Autodesk Inventor part; units mm, degrees
ref_plane "YZ Plane" through (0, 0, 0) normal (1, 0, 0) x (0, 1, 0)
ref_plane "XZ Plane" through (0, 0, 0) normal (0, 1, 0) x (-1, 0, 0)
ref_plane "XY Plane" through (0, 0, 0) normal (0, 0, 1) x (1, 0, 0)
sketch "Sketch1" plane through (0, 0, 0) normal (0, 0, 1) x (1, 0, 0)
  line L0 (0, 0) -> (160, 0)
  line L1 (160, 0) -> (118.589, 154.5481)
  line L2 (41.411, 154.5481) -> (0, 0)
  line L3 (41.411, 154.5481) -> (118.589, 154.5481)
  dimension "d0" = 160
  dimension "d1" = 160
  dimension "d2" = 75
  dimension "d8" = 75
extrude "Extrusion1" add sketch "Sketch1" along normal blind 55
sketch "Sketch7" plane through (0, 0, 0) normal (0, 0, -1) x (-1, 0, 0)
  circle A0 centre (-80, 304.672) radius 315 construction
  line L0 (0, 0) -> (-160, 0)
  arc A1 (-160, 0) -> (0, 0) centre (-80, 304.672) ccw
  dimension "d28" = 630
extrude "Extrusion6" add sketch "Sketch7" against normal blind 55
sketch "Sketch19" plane through (0, 0, 0) normal (0, 0, -1) x (-1, 0, 0)
  circle A0 centre (-80, 4.836) radius 10
  line L0 (-118.589, 154.5481) -> (-41.411, 154.5481)
  line L1 (-80, 154.5481) -> (-80, -10.328)
  arc A1 (-160, 0) -> (0, 0) centre (-80, 304.672) ccw
  dimension "d112" = 20
  dimension "d113" = 15.164
extrude "Extrusion19" cut sketch "Sketch19" against normal through all
sketch "Sketch20" plane through (0, 0, 0) normal (0, 0, -1) x (-1, 0, 0)
  line L0 (-41.411, 154.5481) -> (0, 0)
  circle A0 centre (-80, 4.836) radius 10
  line L1 (-41.411, 154.5481) -> (0, 0)
  line L2 (-118.589, 154.5481) -> (-41.411, 154.5481)
  line L3 (-160, 0) -> (-118.589, 154.5481)
  arc A1 (-160, 0) -> (0, 0) centre (-80, 304.672) ccw
  line L4 (-49.0843, 144.5481) -> (-12.3033, 7.2797)
  arc A2 (-147.6967, 7.2797) -> (-12.3033, 7.2797) centre (-80, 304.672) ccw
  line L5 (-147.6967, 7.2797) -> (-110.9157, 144.5481)
  line L6 (-110.9157, 144.5481) -> (-49.0843, 144.5481)
  line L7 (-15.6678, 19.836) -> (-144.3322, 19.836)
  dimension "d116" = 10
  dimension "d119" = 15
extrude "Extrusion20" cut sketch "Sketch20" against normal through all contours L5 L6 L4 L7
sketch "Sketch21" plane through (0, 0, 0) normal (0, 0, -1) x (-1, 0, 0)
  line L0 (-110.9157, 144.5481) -> (-49.0843, 144.5481)
  line L1 (-75, 144.5481) -> (-75, 19.836)
  line L2 (-15.6678, 19.836) -> (-144.3322, 19.836)
  line L3 (-85, 19.836) -> (-85, 144.5481)
  line L4 (-85, 144.5481) -> (-75, 144.5481)
  line L5 (-75, 19.836) -> (-85, 19.836)
  point P0 (0, 0)
  point P1 (-80, 144.5481)
  point P2 (-80, 144.5481)
  dimension "d120" = 10
extrude "Extrusion21" add sketch "Sketch21" against normal blind 55
sketch "Sketch22" plane through (0, 0, 0) normal (0, 0, -1) x (-1, 0, 0)
  line L0 (-15.6678, 19.836) -> (-49.0843, 144.5481)
  line L1 (-33.7158, 87.1921) -> (-126.2842, 87.1921)
  line L2 (-110.9157, 144.5481) -> (-144.3322, 19.836)
  line L3 (-80, 87.1921) -> (-80, 77.1921)
  line L4 (-31.0363, 77.1921) -> (-128.9637, 77.1921)
  line L5 (-75, 19.836) -> (-75, 144.5481)
  line L6 (-33.7158, 87.1921) -> (-31.0363, 77.1921)
  line L7 (-126.2842, 87.1921) -> (-128.9637, 77.1921)
  point P0 (0, 0)
  point P1 (-80, 82.1921)
  point P2 (-75, 82.1921)
  dimension "d124" = 10
extrude "Extrusion22" add sketch "Sketch22" against normal blind 55
sketch "Sketch23" plane through (0, 0, 0) normal (0, 0, -1) x (-1, 0, 0)
  circle A0 centre (-80, 60) radius 55
  line L0 (-118.589, 154.5481) -> (-41.411, 154.5481)
  line L1 (-57.5, 82.5) -> (-102.5, 82.5)
  line L2 (-102.5, 82.5) -> (-102.5, 37.5)
  line L3 (-102.5, 37.5) -> (-57.5, 37.5)
  line L4 (-57.5, 37.5) -> (-57.5, 82.5)
  point P0 (0, 0)
  point P1 (-80, 154.5481)
  point P2 (-102.5, 60)
  point P3 (-80, 82.5)
  dimension "d127" = 110
  dimension "d128" = 60
  dimension "d129" = 45
  dimension "d130" = 45
extrude "Extrusion23" cut sketch "Sketch23" against normal blind 30 contours L4 L3 L2 L1
sketch "Sketch24" plane through (118.589, 154.5481, 55) normal (0.9659, 0.2588, 0) x (0, 0, -1)
  line L0 (45.475, -9.525) -> (45.475, -150.475) construction
  line L1 (9.525, -150.475) -> (9.525, -9.525) construction
  line L2 (0, -160) -> (0, 0) construction
  circle A0 centre (45.475, -150.475) radius 2.5
  circle A1 centre (9.525, -150.475) radius 2.5
  circle A2 centre (9.525, -9.525) radius 2.5
  circle A3 centre (45.475, -9.525) radius 2.5
  circle A4 centre (18.4199, -150.475) radius 2.5
  circle A5 centre (36.5801, -150.475) radius 2.5
  circle A6 centre (36.5801, -9.525) radius 2.5
  circle A7 centre (18.4199, -9.525) radius 2.5
  point P0 (55, -118.589)
  point P1 (9.525, -80)
  point P2 (0, -80)
  dimension "d133" = 140.95
  dimension "d134" = 140.95
  dimension "d135" = 9.525
  dimension "d136" = 9.525
  dimension "d137" = 5
  dimension "d138" = 5
  dimension "d139" = 5
  dimension "d140" = 5
  dimension "d141" = 5
  dimension "d142" = 5
  dimension "d143" = 5
  dimension "d144" = 5
  dimension "d145" = 18.4199
  dimension "d146" = 18.4199
extrude "Extrusion24" cut sketch "Sketch24" against normal blind 25
sketch "Sketch25" plane through (41.411, 154.5481, 0) normal (-0.9659, 0.2588, 0) x (0, 0, 1)
  line L0 (45.475, -9.525) -> (45.475, -150.475) construction
  line L1 (9.525, -150.475) -> (9.525, -9.525) construction
  circle A0 centre (45.475, -150.475) radius 2.5
  circle A1 centre (9.525, -150.475) radius 2.5
  circle A2 centre (9.525, -9.525) radius 2.5
  circle A3 centre (45.475, -9.525) radius 2.5
  circle A4 centre (18.4199, -150.475) radius 2.5
  circle A5 centre (36.5801, -150.475) radius 2.5
  circle A6 centre (36.5801, -9.525) radius 2.5
  circle A7 centre (18.4199, -9.525) radius 2.5
  line L2 (0, 0) -> (0, -160)
  line L3 (55, 0) -> (55, -160)
  point P0 (9.525, -80)
  point P1 (0, -80)
  dimension "d149" = 140.95
  dimension "d150" = 140.95
  dimension "d153" = 5
  dimension "d154" = 5
  dimension "d155" = 5
  dimension "d156" = 5
  dimension "d157" = 5
  dimension "d158" = 5
  dimension "d159" = 5
  dimension "d160" = 5
  dimension "d163" = 9.525
  dimension "d164" = 18.4199
  dimension "d165" = 18.4199
  dimension "d166" = 9.525
extrude "Extrusion25" cut sketch "Sketch25" against normal blind 25
properties part number "CA001" material "ABS Plastic"
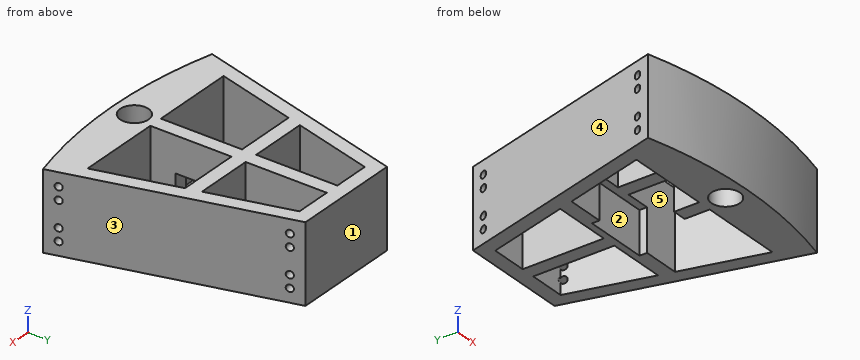
Model file for the job. Use its own axes, mm. Face numbers are marked on the shaded views. A direction names the side the tool comes from. Coordinates: 2 decimals unless noted, no trailing zeros. Write each loop counter-clockwise with the first axis right and the second up, starting at its lowest first coordinate (ties: lowest second). Pieces come first, ordered by that corner, then holes. Notation, with made-up numbers: (46.25, 0) - (55.25, 0) arc R23 cw to (55.25, 27) - close; hole circle Ø7 at (11, -40). An arc over 180 degrees is marked (long way). One line per item, written item: value. Start each with the question number.
1. Mould opens along X. For the marked faces 1, 2 and 3 say: released by +X, released by -X, zero draft, split by the parting line, or undercut.
2. Slice it at A-A (x = 80). Write the cut outline in (y, z), plus the area to 3 significant figures.
3. Slice it at D-D (x = 105.5). Write the cut outline in (y, z), plus the area to 3 significant figures.
4. Flat gauge pins, fed straight in: pin 1 (1.5 mm diameter, centred on y = 31.5, z = 29, fed in from -X); pin 2 (4 mm diameter, centred on x = 108, y = 18, fed in from -Z); pin 3 (6 mm diameter, centred on y = 59, z = 17.5, fed in from -X); pin 4 (13 mm diameter, centred on x = 97, z = 39, fed in from -Y). Where does each tip first touch, or does it go through?
5. Slice it at B-B (y = 47). Write the cut outline in (x, z).
6. Slice it at C-C (z = 4). Write the cut outline in (x, y).
7. Tool access for the marked faces 4 and 5: list every direction of +Z, -Z, +X, -X, +Y, -Y with a clear straight run to the whole face (end or side of a thin tool).
8. Probe line 1 (Y direction, x = 80, z = 17); line 2 (Y direction, x = 80, z = 34); line 3 (X direction, y = 109, z = 42). List the from-to ranges inside material, lowest first. Write a range as from..to.
Answers below:
1. face 1: zero draft
1. face 2: undercut
1. face 3: released by +X
2. outline: (-10.33, 0) - (-5.16, 0) - (-5.16, 55) - (-10.33, 55) - close; (14.84, 0) - (37.5, 0) - (37.5, 30) - (82.5, 30) - (82.5, 0) - (154.55, 0) - (154.55, 55) - (14.84, 55) - close
2. area: 6,620 mm^2
3. outline: (-9.29, 0) - (19.84, 0) - (19.84, 55) - (-9.29, 55) - close; (77.19, 0) - (87.19, 0) - (87.19, 55) - (77.19, 55) - close; (144.55, 0) - (154.55, 0) - (154.55, 55) - (144.55, 55) - close
3. area: 2,700 mm^2
4. pin 1: stops at x = 8.24
4. pin 2: stops at z = 0
4. pin 3: stops at x = 15.01
4. pin 4: stops at y = -10.15
5. outline: (12.59, 0) - (22.95, 0) - (22.95, 55) - (12.59, 55) - close; (75, 30) - (85, 30) - (85, 55) - (75, 55) - close; (137.05, 0) - (147.41, 0) - (147.41, 55) - (137.05, 55) - close
6. outline: (0, 0) arc R315 ccw to (160, 0) - (118.59, 154.55) - (41.41, 154.55) - close; hole (15.67, 19.84) - (75, 19.84) - (75, 37.5) - (85, 37.5) - (85, 19.84) - (144.33, 19.84) - (128.96, 77.19) - (102.5, 77.19) - (102.5, 82.5) - (57.5, 82.5) - (57.5, 77.19) - (31.04, 77.19) - close; hole (33.72, 87.19) - (75, 87.19) - (75, 144.55) - (49.08, 144.55) - close; hole circle Ø20 at (80, 4.84); hole (85, 87.19) - (126.28, 87.19) - (110.92, 144.55) - (85, 144.55) - close
7. face 4: +Z, -Z, -X, +Y
7. face 5: +Z, -Z
8. line 1: y = -10.33..-5.16, 14.84..37.5, 82.5..154.55
8. line 2: y = -10.33..-5.16, 14.84..154.55
8. line 3: x = 29.21..39.56, 75..85, 120.44..130.79
